The drawing under review shows one solid part. Ordinate dimensions are in mm from its lowest x, y, z. A direction names the side the tool comes from. Round coordinates to 2 decimals unless told otherwise and drop trailing zeros. Write each loop counter-clockwise with the first axis right and the second up, starting at its lowest first coordinate (ties: lowest second). Pieces come first, ordered by that corner, then holes.
Item 1: Add section D-D (x = 5). Give the boundary of the cut face in (y, z), plus the area to 3 significant figures.
Item 2: Draft analysis for pull direction Y (two halves, no side actions). For the marked faces 1, 2 and 3, state which applies: +Y half, -Y half, draft (parallel to the pull), parting line (faces both ways), or undercut.
Item 3: To check wall thickness, follow L1, parallel to Y at x = 2.75, z = 17.5; L2, parallel to X at y = 4.75, z = 19; L3, parallel to Z at x = 3.5, y = 7.5. State the ranges of each line that lie inside material, in increasing order.
Item 4: Machinability: for the marked faces 4, 5 and 6, which of the approach directions +Z, -Z, +X, -X, +Y, -Y give a long, thin tool a straight path to every point of the face, cutting with its end or side? Answer none if there is none.
Item 5: Clearance check with flat-ended pins moving along their axes: pin 1 Ø4 at (x, z) = (4.5, 10) entering from -Y (3 decimals); pin 2 Ø4 at (y, z) = (3.5, 11.5) entering from -X. State where each tip first meets the part, or that it passes through.
Item 6: Add section A-A (y = 3.95). Give the boundary of the cut face in (x, z).
Item 7: Add section B-B (z = 16.5). Give the boundary of the cut face in (x, y).
Item 8: Add section C-C (y = 1.25). Give the boundary of the cut face in (x, z), plus the area to 4 significant figures.
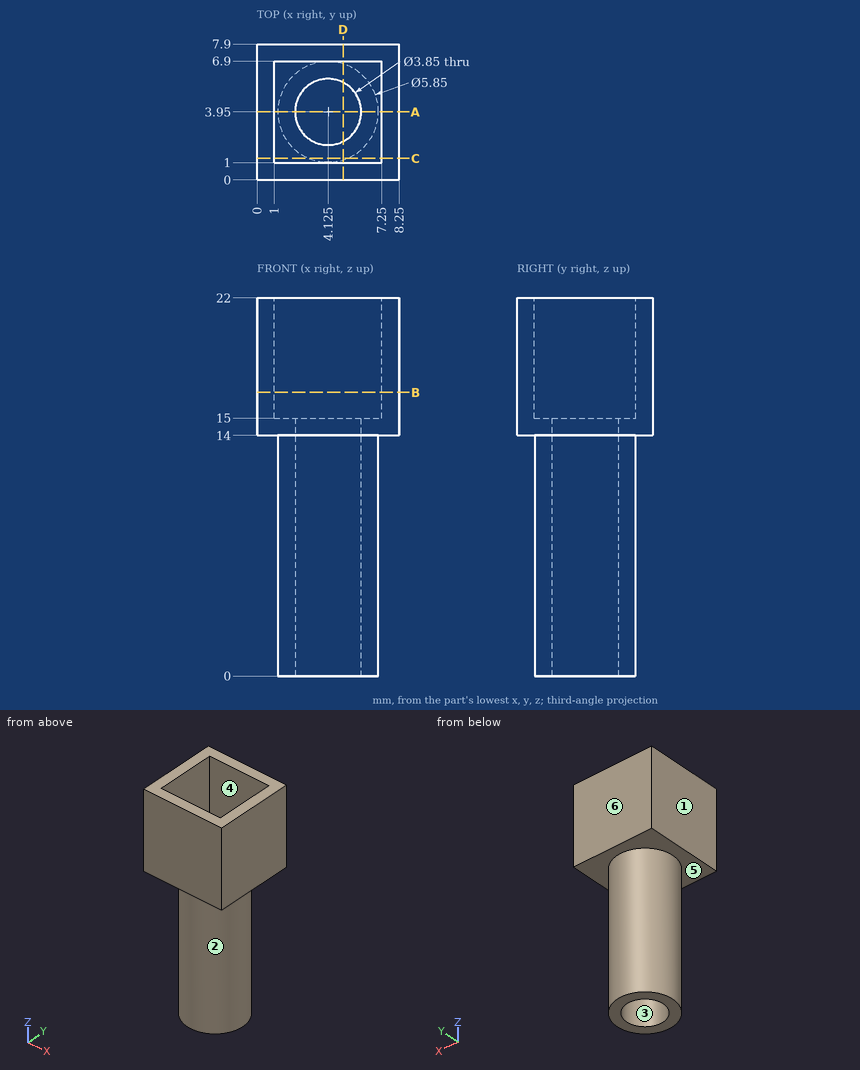
Numbers:
1. outline: (0, 14) - (1.16, 14) - (1.16, 0) - (2.24, 0) - (2.24, 15) - (1, 15) - (1, 22) - (0, 22) - close; (5.66, 0) - (6.74, 0) - (6.74, 14) - (7.9, 14) - (7.9, 22) - (6.9, 22) - (6.9, 15) - (5.66, 15) - close
1. area: 48.6 mm2
2. face 1: draft
2. face 2: parting line
2. face 3: undercut
3. L1: y = 0 to 1, 6.9 to 7.9
3. L2: x = 0 to 1, 7.25 to 8.25
3. L3: z = 14 to 22
4. face 4: +Z
4. face 5: -Z
4. face 6: +Z, -Z, +X, -X, +Y
5. pin 1: stops at y = 1.025
5. pin 2: stops at x = 1.2
6. outline: (0, 14) - (1.2, 14) - (1.2, 0) - (2.2, 0) - (2.2, 15) - (1, 15) - (1, 22) - (0, 22) - close; (6.05, 0) - (7.05, 0) - (7.05, 14) - (8.25, 14) - (8.25, 22) - (7.25, 22) - (7.25, 15) - (6.05, 15) - close
7. outline: (0, 0) - (8.25, 0) - (8.25, 7.9) - (0, 7.9) - close; hole (1, 1) - (7.25, 1) - (7.25, 6.9) - (1, 6.9) - close
8. outline: (0, 14) - (3, 14) - (3, 0) - (5.25, 0) - (5.25, 14) - (8.25, 14) - (8.25, 22) - (7.25, 22) - (7.25, 15) - (1, 15) - (1, 22) - (0, 22) - close
8. area: 53.75 mm2
